Could you check a few things on this drawing? It's one solid part, dimensions in mm from its lowest x, y, z. A direction names the side the tool comes from. Give positions to 0.01 mm unless a question says otherwise; leave off trailing zeros. Order: outer loops, then holes, each group sorted by start corner. A loop starts at its lowest first (then second) coordinate and runs counter-clockwise, first axis right, second up.
Item 1: I want a section at A-A, the plane z = 148. Write out the boundary of the cut face in (x, y) (1 decimal), then the cut area to 3 significant figures.
Item 2: Which directions (+Z, -Z, +X, -X, +Y, -Y) give clear straight access to the entire face, cutting with the end or side of a thin tool? Please do the marked faces 3, 4 and 5.
Item 3: If I drill on line 1 along X through (y, z) = (41, 17); line 2 along X through (y, z) = (34.5, 148) (1 decimal); line 3 along Y through (x, z) = (25, 214), over which ranges is the centre line in solid material (lowest first)?
Item 4: I'm going to push flat-ended pins straight in: pin 1 Ø8 at (x, z) = (42, 209.5) entering from -Y; pin 2 Ø6 at (y, z) = (85, 123) entering from -X (1 decimal); pin 3 Ø11.5 at (x, y) = (56.5, 41) entering from -Z; pin 4 Ø5 at (x, y) = (80, 73) entering from +Z. Where does each tip first touch, or does it pass through?
Item 5: I want a section at B-B, the plane z = 284. Write out the boundary of the cut face in (x, y) (1 decimal), then the cut area to 3 significant figures.
Item 6: If we mould it in two halves opening along X, with no side actions, what happens to the marked faces 1 and 2? For each: +X half, -X half, draft (parallel to the pull), parting line (faces both ways), or undercut.
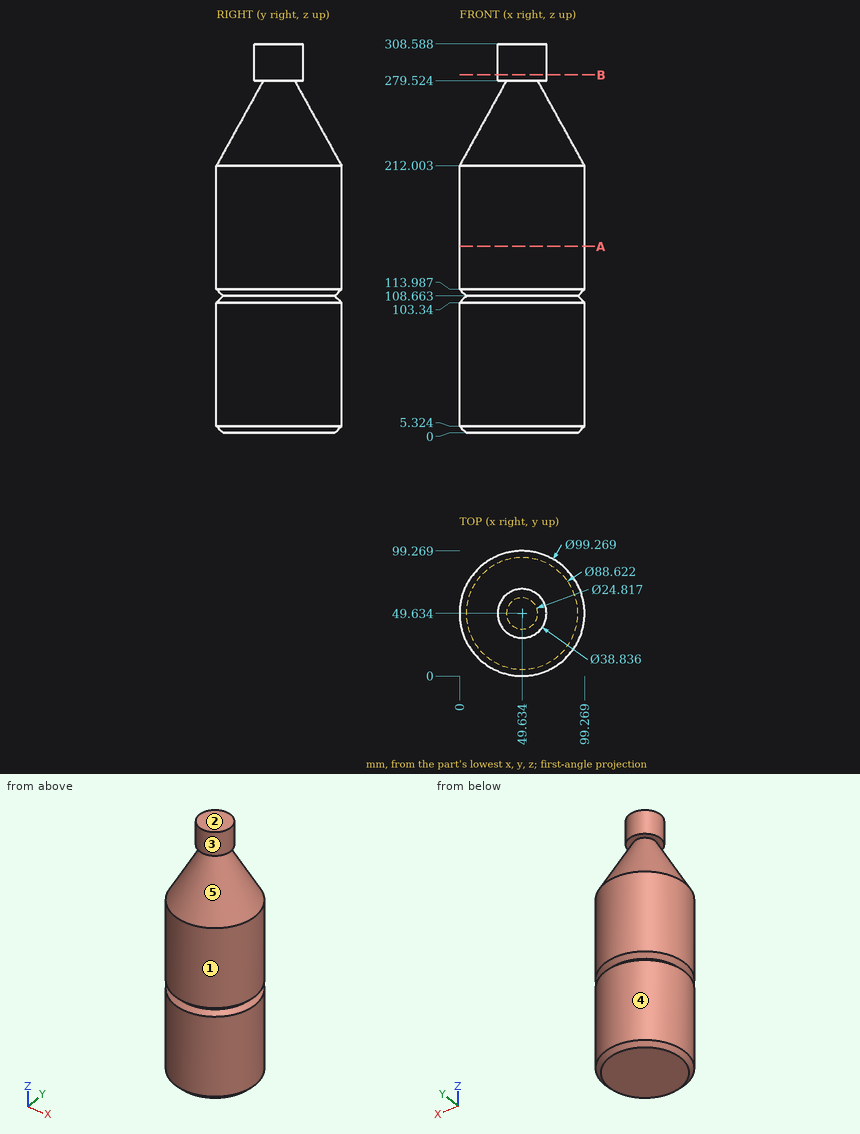
Results list:
1. outline: circle Ø99.3 at (49.6, 49.6)
1. area: 7,740 mm2
2. face 3: +Z
2. face 4: +Z, -Z
2. face 5: none
3. line 1: x = 0.76 to 98.51
3. line 2: x = 2.4 to 96.9
3. line 3: y = 7.82 to 91.45
4. pin 1: stops at y = 0.13
4. pin 2: stops at x = 12
4. pin 3: stops at z = 0
4. pin 4: stops at z = 237.07
5. outline: circle Ø38.8 at (49.6, 49.6)
5. area: 1,180 mm2
6. face 1: parting line
6. face 2: draft
